Answer from the drawing. Dimensions are ordinates in mm from the lowest x, y and z of the part. Coordinates: 2 decimals unless noted, no trailing zeros. Order: outer loops, then holes, each group sorted by start corner. A loop starts at its lowest first (then second) coordinate and runs counter-clockwise, first axis right, second up. Notation, with made-up numbers: (54, 71) -> (68, 71) arc R33 cw to (68, 106) -> close; hole circle Ø6 at (-15, 44). An arc over 180 degrees is marked (long way). Answer in a Markdown table with one row per item.
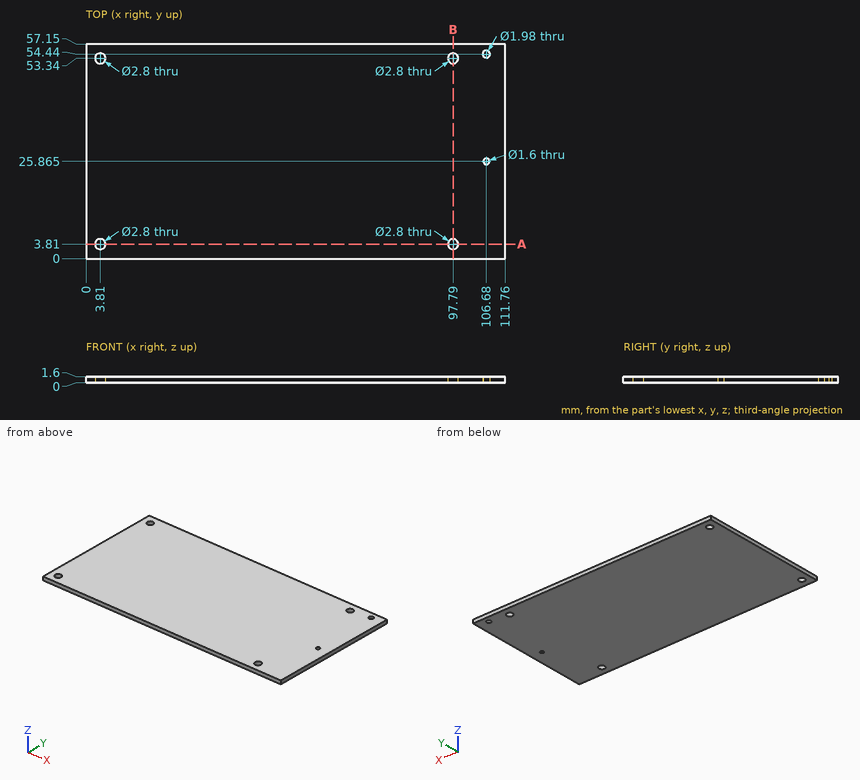
Q1. Consider line 1 (Y direction, x = 106.5, z = 0.5); line 2 (Y direction, x = 3.81, z = 0.8). Determine where each line is inside the solid, lowest interval first.
Outcome:
| item | result |
|---|---|
| line 1 | 0 to 25.09, 26.64 to 53.47, 55.41 to 57.15 |
| line 2 | 0 to 2.41, 5.21 to 51.94, 54.74 to 57.15 |
Q2. The part is cut by section B-B (x = 97.79). Write down the section's boundary in (y, z).
Outcome:
| item | result |
|---|---|
| outline | (0, 0) -> (2.41, 0) -> (2.41, 1.6) -> (0, 1.6) -> close; (5.21, 0) -> (51.94, 0) -> (51.94, 1.6) -> (5.21, 1.6) -> close; (54.74, 0) -> (57.15, 0) -> (57.15, 1.6) -> (54.74, 1.6) -> close |
Q3. The part is cut by section A-A (y = 3.81). Write down the section's boundary in (x, z), then the cut area to 3 significant figures.
Outcome:
| item | result |
|---|---|
| outline | (0, 0) -> (2.41, 0) -> (2.41, 1.6) -> (0, 1.6) -> close; (5.21, 0) -> (96.39, 0) -> (96.39, 1.6) -> (5.21, 1.6) -> close; (99.19, 0) -> (111.76, 0) -> (111.76, 1.6) -> (99.19, 1.6) -> close |
| area | 170 mm² |
